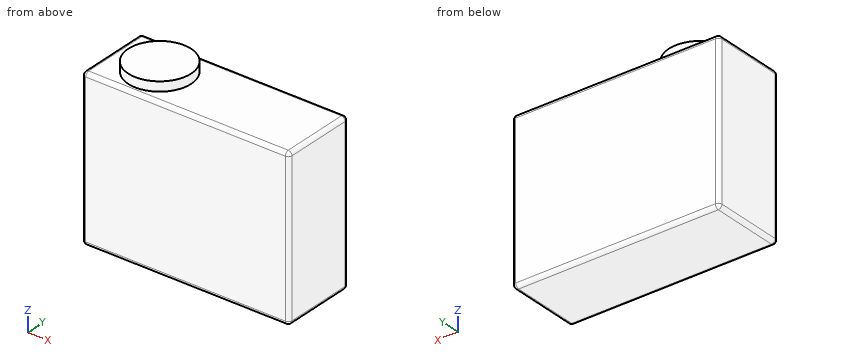
from build123d import *

# Parameters (mm, degrees)
F0_W     = 275
F0_H     = 210
F1_DEPTH = 100
F2_R     = 5
F3_R     = 41.712108
F4_DEPTH = 12.5


with BuildPart() as f1:
    # F0 (on Front) → F1 (new body)
    with BuildSketch(Plane.XZ):
        Rectangle(F0_W, F0_H)
    extrude(amount=F1_DEPTH)

    # F2
    f2_edges = [f1.edges().sort_by_distance(p)[0] for p in [
        (-137.5, -50, 105),
        (-137.5, -50, -105),
        (-137.5, 0, 0),
        (-137.5, -100, 0),
        (137.5, -50, 105),
        (0, 0, 105),
        (0, -100, 105),
        (0, 0, -105),
        (137.5, 0, 0),
        (137.5, -50, -105),
        (137.5, -100, 0),
        (0, -100, -105),
    ]]
    fillet(f2_edges, radius=F2_R)

    # F3 (on face) → F4 (join)
    with BuildSketch(Plane.XY.offset(105)):
        with Locations((-73.406562, -50)):
            Circle(F3_R)
    extrude(amount=F4_DEPTH)


solid = f1.part
Check sheet for the modelled part. Datum: model origin and axes. Units: mm. Coordinates: 2 decimals unless noted, no trailing zeros. Loops run counter-clockwise (first coordinate to the right, second up) from the corner with the lowest first, then second, coordinate; pieces in that order, holes last. Notation, with made-up numbers: (81.25, 84) -> (104.25, 84) arc R9 cw to (104.25, 99) -> close; hole circle Ø6 at (41.25, 26.5). An arc over 180 degrees is marked (long way). Answer in a Markdown table with one row per item.
1. Sectioned sample at B-B, the plane y = -50. Record the boundary of the cut face in (x, z).
Check values:
| item | result |
|---|---|
| outline | (-137.5, -100) arc R5 ccw to (-132.5, -105) -> (132.5, -105) arc R5 ccw to (137.5, -100) -> (137.5, 100) arc R5 ccw to (132.5, 105) -> (-31.69, 105) -> (-31.69, 117.5) -> (-115.12, 117.5) -> (-115.12, 105) -> (-132.5, 105) arc R5 ccw to (-137.5, 100) -> close |
2. Sectioned sample at C-C, the plane x = -51. Record the boundary of the cut face in (y, z), then the cut area to 3 significant figures.
Check values:
| item | result |
|---|---|
| outline | (-100, -100) arc R5 ccw to (-95, -105) -> (-5, -105) arc R5 ccw to (0, -100) -> (0, 100) arc R5 ccw to (-5, 105) -> (-14.82, 105) -> (-14.82, 117.5) -> (-85.18, 117.5) -> (-85.18, 105) -> (-95, 105) arc R5 ccw to (-100, 100) -> close |
| area | 21,900 mm2 |
3. Sectioned sample at A-A, the plane x = 35. Record the boundary of the cut face in (y, z), then the cut area to 3 significant figures.
Check values:
| item | result |
|---|---|
| outline | (-100, -100) arc R5 ccw to (-95, -105) -> (-5, -105) arc R5 ccw to (0, -100) -> (0, 100) arc R5 ccw to (-5, 105) -> (-95, 105) arc R5 ccw to (-100, 100) -> close |
| area | 21,000 mm2 |
4. Go/stop test with a flat-tipped pin: pin 1 (12 mm diameter, centred on x = 90.5, y = -26, fed in from +Z). Record where the tip stops, or that it passes through.
Check values:
| item | result |
|---|---|
| pin 1 | stops at z = 105 |
5. Material ranges on line 1 along Z through (x, y) = (-20.5, -17.5); line 2 along X through (y, z) = (-27.5, 105.5), recorded low to high. Write a range as [from, to].
Check values:
| item | result |
|---|---|
| line 1 | z = [-105, 105] |
| line 2 | x = [-108.53, -38.28] |
